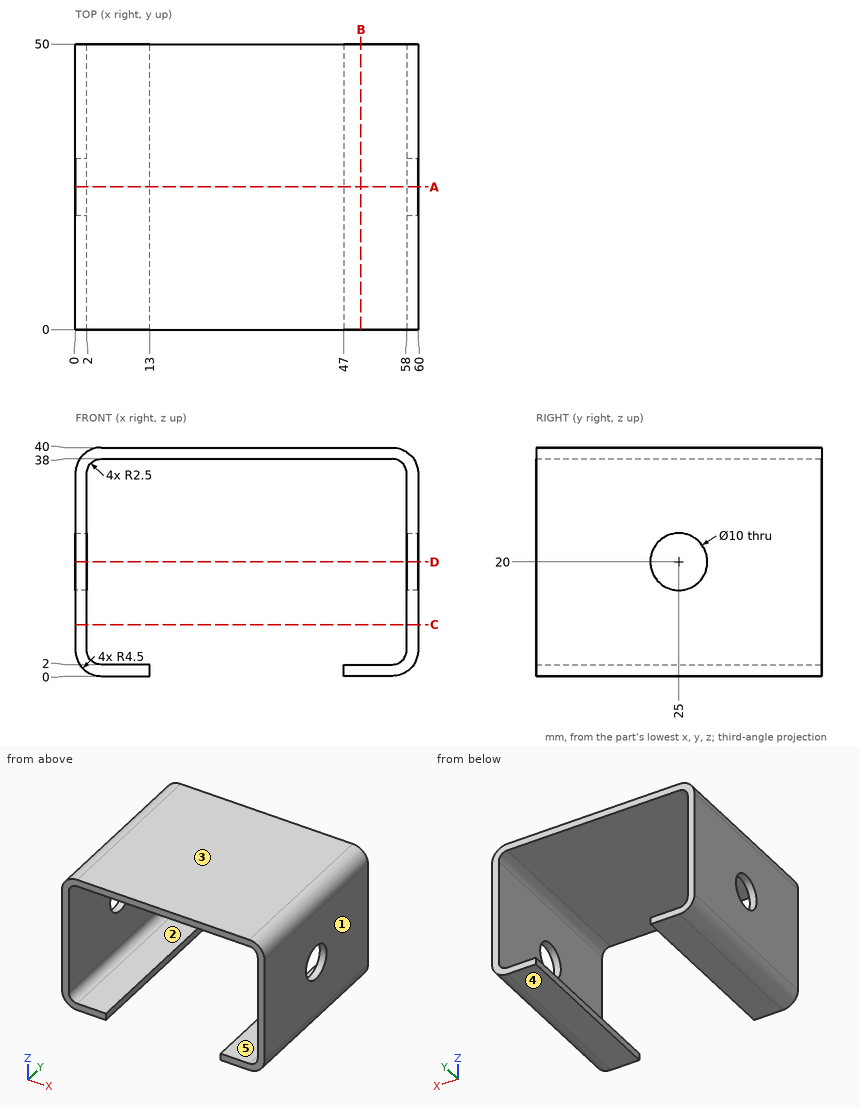
Design review of the part shown in the three views and the two pictorial views. Dimensions are in mm from the part's minimum x, y and z. A direction names the side the tool comes from. Give positions to 0.01 mm unless a question says otherwise; leave off trailing zeros. Write each loop counter-clockwise with the first axis right and the second up, starting at its lowest first coordinate (ties: lowest second). Pieces come first, ordered by that corner, then holes.
Item 1: Take a section at B-B (x = 50). Give the boundary of the cut face in (y, z).
Item 2: Take a section at D-D (z = 20). Give the boundary of the cut face in (x, y), and give its area (3 significant figures).
Item 3: Take a section at A-A (y = 25). Give the boundary of the cut face in (x, z), and give its area (3 significant figures).
Item 4: The part is to be moulded in two halves that separate along Z. For the marked faces 3, 4 and 5, say which applies: +Z half, -Z half, draft (parallel to the pull), parting line (faces both ways), or undercut.
Item 5: Wall thickness on probe 1 along X at (y, z) = (32, 29); probe 2 along Z at (x, y) = (8, 13); probe 3 along Y at (x, z) = (0.7, 20): over which ranges is each line inside the solid? List them lowest first.
Item 6: Take a section at C-C (z = 9). Give the boundary of the cut face in (x, y), and give its area (3 significant figures).
Item 7: Machinability: for the marked faces 1 and 2, which of the approach directions +Z, -Z, +X, -X, +Y, -Y give a long, thin tool a straight path to every point of the face, cutting with its end or side? Answer none if there is none.
Item 8: Insertion check: P1, Ø2, axis at y = 23, z = 1.5, coming from the -X side; P2, Ø1.5, axis at x = 16.5, y = 23, coming from the -Z side; P3, Ø2, axis at y = 33.5, z = 1.5, coming from the +X side. Each pin has a flat end and moves straight along its axis. Give the tip position at first contact, or say it passes through.
Established:
1. outline: (0, 0) - (50, 0) - (50, 2) - (0, 2) - close; (0, 38) - (50, 38) - (50, 40) - (0, 40) - close
2. outline: (0, 0) - (2, 0) - (2, 20) - (0, 20) - close; (0, 30) - (2, 30) - (2, 50) - (0, 50) - close; (58, 0) - (60, 0) - (60, 20) - (58, 20) - close; (58, 30) - (60, 30) - (60, 50) - (58, 50) - close
2. area: 160 mm2
3. outline: (0, 4.5) arc R4.5 ccw to (4.5, 0) - (13, 0) - (13, 2) - (4.5, 2) arc R2.5 cw to (2, 4.5) - (2, 15) - (0, 15) - close; (0, 25) - (2, 25) - (2, 35.5) arc R2.5 cw to (4.5, 38) - (55.5, 38) arc R2.5 cw to (58, 35.5) - (58, 25) - (60, 25) - (60, 35.5) arc R4.5 ccw to (55.5, 40) - (4.5, 40) arc R4.5 ccw to (0, 35.5) - close; (47, 0) - (55.5, 0) arc R4.5 ccw to (60, 4.5) - (60, 15) - (58, 15) - (58, 4.5) arc R2.5 cw to (55.5, 2) - (47, 2) - close
3. area: 264 mm2
4. face 3: +Z half
4. face 4: -Z half
4. face 5: undercut
5. probe 1: x = 0 to 2, 58 to 60
5. probe 2: z = 0 to 2, 38 to 40
5. probe 3: y = 0 to 20, 30 to 50
6. outline: (0, 0) - (2, 0) - (2, 50) - (0, 50) - close; (58, 0) - (60, 0) - (60, 50) - (58, 50) - close
6. area: 200 mm2
7. face 1: +Z, -Z, +X, +Y, -Y
7. face 2: +Y, -Y
8. P1: stops at x = 0.47
8. P2: stops at z = 38
8. P3: stops at x = 59.53
